Autodesk Inventor part; units mm, degrees
ref_plane "YZ Plane" through (0, 0, 0) normal (1, 0, 0) x (0, 1, 0)
ref_plane "XZ Plane" through (0, 0, 0) normal (0, 1, 0) x (-1, 0, 0)
ref_plane "XY Plane" through (0, 0, 0) normal (0, 0, 1) x (1, 0, 0)
sketch "スケッチ1" plane through (0, 0, 0) normal (0, 1, 0) x (-1, 0, 0)
  circle A0 centre (0, 0) radius 52
  line L0 (27.9396, 43.8564) -> (27.9396, -43.8564)
  line L1 (27.9396, -43.8564) -> (0, 0)
  line L2 (0, 0) -> (52, 0)
  line L3 (27.9396, 43.8564) -> (0, 0)
  line L4 (0, 52) -> (0, -52)
  line L5 (-27.9396, 43.8564) -> (-27.9396, -43.8564)
  line L6 (-27.9396, -43.8564) -> (0, 0)
  line L7 (-27.9396, 43.8564) -> (0, 0)
  dimension "d0" = 104
  dimension "d1" = 57.5
extrude "押し出し1" add sketch "スケッチ1" along normal blind 18.35 contours L3 L4 A0 | L0 L2 L3 | L1 L2 L0 | A0 L4 L1 | L4 L7 A0 | L4 A0 L6 | L6 L5 L7
sketch "スケッチ2" plane through (0, 18.35, 0) normal (0, 1, 0) x (1, 0, 0)
  circle A0 centre (0, 0) radius 39.9
  dimension "d4" = 79.8
extrude "押し出し2" cut sketch "スケッチ2" against normal blind 14.6
sketch "スケッチ3" plane through (0, 0, 0) normal (0, -1, 0) x (1, 0, 0)
  line L0 (0, 0) -> (0, 52)
  arc A0 (27.9396, 43.8564) -> (-27.9396, 43.8564) centre (0, 0) ccw
  line L1 (0, 0) -> (19.8995, 48.0417)
  line L2 (0, 0) -> (27.9396, 0)
  line L3 (27.9396, -28.4849) -> (27.9396, 28.4849)
  point P0 (18.7515, 45.2701)
  point P1 (-18.7515, 45.2701)
  point P2 (18.7515, -45.2701)
  point P3 (-18.7515, -45.2701)
  dimension "d8" = 98
  dimension "d7" = 22.5
hole "穴1" at (18.7515, 0, 45.2701) at (-18.7515, 0, 45.2701) at (-18.7515, 0, -45.2701) at (18.7515, 0, -45.2701) direction (0, 1, 0) diameter 4.2 end through all
fillet "フィレット1" radius 1 16 edges at (0, 18.35, 39.9) (0, 18.35, -39.9) (0, 18.35, 52) (27.9396, 3.75, 0) (27.9396, 0, 0) (27.9396, 11.05, 28.4849) (27.9396, 11.05, -28.4849) (27.9396, 9.175, 43.8564) (-27.9396, 9.175, 43.8564) (-27.9396, 11.05, 28.4849) (-27.9396, 11.05, -28.4849) (27.9396, 9.175, -43.8564) (0, 18.35, -52) (-27.9396, 9.175, -43.8564) (-27.9396, 3.75, 0) (-27.9396, 0, 0)
properties part number "base_part8"
Input: part model. Units: mm. Frame: model coordinates. A direction names the side the tool comes from. Coordinates: 2 decimals unless noted, no trailing zeros. Loops run counter-clockwise (first coordinate to the right, second up) from the corner with the lowest first, then second, coordinate; pieces in that order, holes last. Notation, with made-up numbers: M 7.25,72 L 30.25,72 A10 ccw 30.25,76 Z; hole C -8.5,69 d5. An arc over 180 degrees is marked long. Use a Markdown table: item, result. Add a question column.
1) Line query: L1, parallel to Z at x = -17, y = 14; L2, parallel to Z at x = 21, y = 10.5; L3, parallel to Y at x = -9.5, z = -37. Output: solid intervals per line, ascending. Write a range as from..to.
2) Draft query along Z for faces 3 (the cylindrical face through (0, 9, -52)), 4 (the cylindrical face through (18.659, 9.303, -43.172)), 5 (the flat face through (27.94, 1.3, 0.2)). Return one class per face: +Z half, -Z half, draft (parallel to the pull), parting line (faces both ways), or undercut.
3) Set-up query: faces 1 (the flat face through (0, 3.75, -1)), 2 (the cylindrical face through (0, 9, 52)). Return all of +Z, -Z, +X, -X, +Y, -Y with unobstructed straight access to the full face (end or side cutting, diameter ignored); none if empty.
4) Section A-A, the plane z = -18. Return the cut outline in (x, y).
5) Pin query (flat end, axial travel): P1, Ø3.5, axis at x = -18.75, z = -45.27, coming from the +Y side; P2, Ø1.5, axis at x = -13, y = 13, coming from the +Z side; P3, Ø5, axis at x = 19.5, y = 15.5, coming from the +Z side; P4, Ø5, axis at x = -19.5, y = 13.5, coming from the -Z side. Return the tip coordinate at first contact, or that it passes through.
6) Section B-B, the plane y = 12.75. Return the cut outline in (x, z), plus the area to 3 significant figures.
Answer below:
| question | item | result |
|---|---|---|
| 1 | L1 | -49.14..-46.43, -44.11..-36.1, 36.1..44.11, 46.43..49.14 |
| 1 | L2 | -47.57..-33.93, 33.93..47.57 |
| 1 | L3 | 0..3.75 |
| 2 | face 3 | -Z half |
| 2 | face 4 | undercut |
| 2 | face 5 | draft |
| 3 | face 1 | +Y |
| 3 | face 2 | +Z, +Y, -Y |
| 4 | outline | M -27.94,1 A1 ccw -26.94,0 L 26.94,0 A1 ccw 27.94,1 L 27.94,2.75 A1 ccw 26.94,3.75 L -26.94,3.75 A1 ccw -27.94,2.75 Z |
| 5 | P1 | through |
| 5 | P2 | z = 50.54 |
| 5 | P3 | z = 49.14 |
| 5 | P4 | z = -49.14 |
| 6 | outline | M -27.94,-43.3 A1 ccw -27.47,-44.15 A52 ccw 27.47,-44.15 A1 ccw 27.94,-43.3 L 27.94,-30.77 A1 ccw 26.28,-30.02 A39.9 cw -26.28,-30.02 A1 ccw -27.94,-30.77 Z; M -27.94,30.77 A1 ccw -26.28,30.02 A39.9 cw 26.28,30.02 A1 ccw 27.94,30.77 L 27.94,43.3 A1 ccw 27.47,44.15 A52 ccw -27.47,44.15 A1 ccw -27.94,43.3 Z; hole C -18.75,-45.27 d4.2; hole C -18.75,45.27 d4.2; hole C 18.75,-45.27 d4.2; hole C 18.75,45.27 d4.2 |
| 6 | area | 1,400 mm2 |
